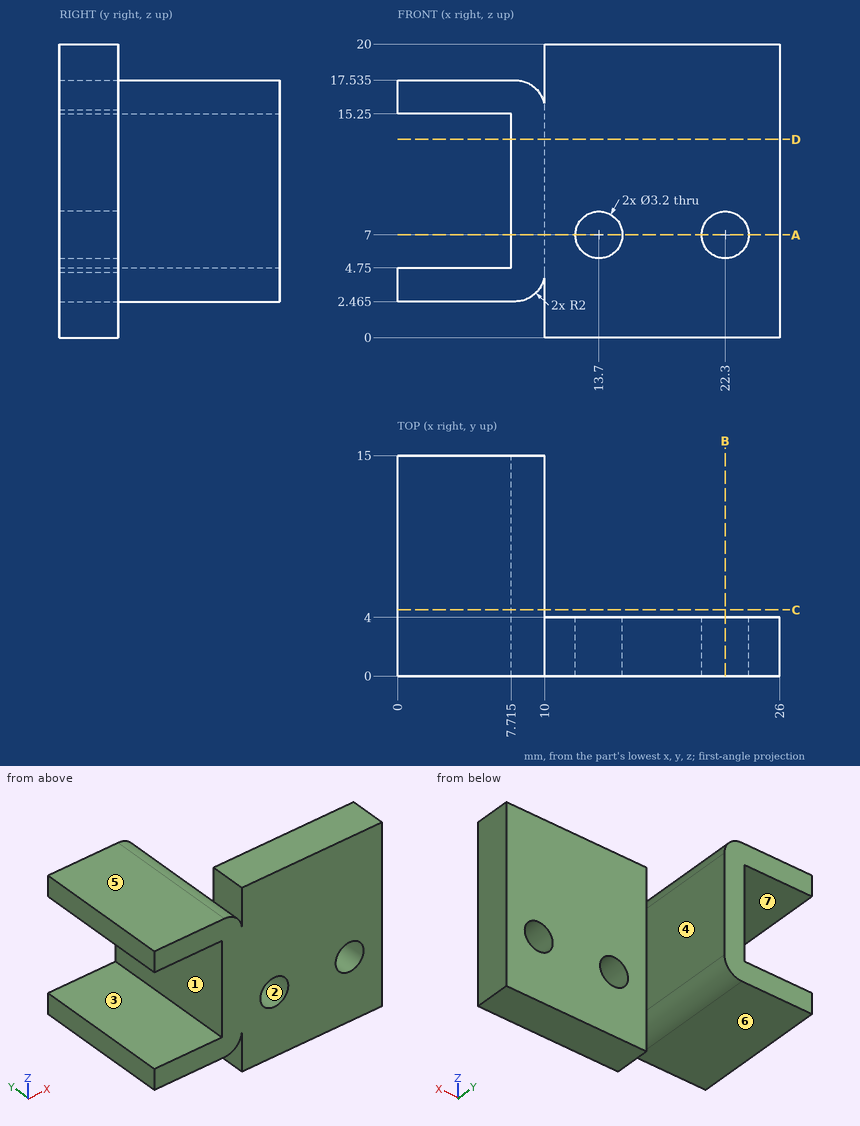
Geometry check sheet. Reference: drawing and pictorial views, mm from the part's lowest x, y, z. A direction names the side the tool comes from. Give positions to 0.01 mm unless a question says otherwise; leave off trailing zeros. Order: outer loops, then holes, each group sorted by start corner. A loop starts at its lowest first (then second) coordinate and runs counter-clockwise, first axis right, second up. Notation, with made-up numbers: M 33.25,-24.75 L 51.25,-24.75 A25 ccw 51.25,-10.75 Z; hole C -28,8.5 d10. An arc over 180 degrees is marked long. Answer in a Markdown table with one row per item. Add a question column.
Item 1: Tool access check on the marked faces 4, 5, 6 and 7. Record the directions out of +Z, -Z, +X, -X, +Y, -Y that give a thin tool (end or side, any length) a straight path to the whole face; none if there is none.
Item 2: Gauge pin test, flat ends, axial feed: pin 1 (3.5 mm diameter, centred on x = 13.7, z = 7, fed in from +Y); pin 2 (4 mm diameter, centred on x = 2.5, y = 8, fed in from -Z) (3 decimals); pin 3 (3 mm diameter, centred on x = 22.3, z = 7, fed in from -Y); pin 4 (3.5 mm diameter, centred on y = 12, z = 12, fed in from +X). Record the tip position at first contact, or that the pin passes through.
Item 3: Mould release check, pull along X, two halves, no side actions. Record for the marked faces 1, 2 and 3: released by +X, released by -X, zero draft, split by the parting line, or undercut.
Item 4: Section check D-D, the plane z = 13.5. Enter the section's corners in (x, y) (3 decimals), and give its area (3 significant figures).
Item 5: Section check A-A, the plane z = 7. Enter the section's corners in (x, y) (3 decimals).
Item 6: Section check B-B, the plane x = 22.3. Enter the section's corners in (y, z), and give its area (3 significant figures).
Item 7: Section check C-C, the plane y = 4.5. Enter the section's corners in (x, z) (3 decimals).
Item 8: Scan lines: probe 1 along X at (y, z) = (2.55, 7) (3 decimals); probe 2 along Z at (x, y) = (6, 6.75) (3 decimals); probe 3 along X at (y, z) = (7.5, 8) (3 decimals). Record each from-to range of solid material in increasing order. Write a range as from..to.
Filled sheet:
| question | item | result |
|---|---|---|
| 1 | face 4 | +Z, -Z, +X, +Y |
| 1 | face 5 | +Z, -X, +Y, -Y |
| 1 | face 6 | -Z, -X, +Y, -Y |
| 1 | face 7 | -X, +Y, -Y |
| 2 | pin 1 | stops at y = 4 |
| 2 | pin 2 | stops at z = 2.465 |
| 2 | pin 3 | passes through |
| 2 | pin 4 | stops at x = 10 |
| 3 | face 1 | released by -X |
| 3 | face 2 | undercut |
| 3 | face 3 | zero draft |
| 4 | outline | M 7.715,0 L 26,0 L 26,4 L 10,4 L 10,15 L 7.715,15 Z |
| 4 | area | 98.3 mm^2 |
| 5 | outline | M 7.715,0 L 12.1,0 L 12.1,4 L 10,4 L 10,15 L 7.715,15 Z; M 15.3,0 L 20.7,0 L 20.7,4 L 15.3,4 Z; M 23.9,0 L 26,0 L 26,4 L 23.9,4 Z |
| 6 | outline | M 0,0 L 4,0 L 4,5.4 L 0,5.4 Z; M 0,8.6 L 4,8.6 L 4,20 L 0,20 Z |
| 6 | area | 67.2 mm^2 |
| 7 | outline | M 0,2.465 L 8,2.465 A2 ccw 10,4.465 L 10,15.535 A2 ccw 8,17.535 L 0,17.535 L 0,15.25 L 7.715,15.25 L 7.715,4.75 L 0,4.75 Z |
| 8 | probe 1 | x = 7.715..12.1, 15.3..20.7, 23.9..26 |
| 8 | probe 2 | z = 2.465..4.75, 15.25..17.535 |
| 8 | probe 3 | x = 7.715..10 |
